Geometry check sheet. Reference: the model listing, model coordinates, mm. Face numbers are marked on the shaded views. A direction names the side the tool comes from. Coordinates: 2 decimals unless noted, no trailing zeros. Order: outer loops, then holes, each group sorted by start corner. A loop starts at its lowest first (then second) coordinate and runs counter-clockwise, first axis right, second up. Notation, with made-up numbers: (32.5, -18) - (63.5, -18) arc R8 cw to (63.5, -14) - close; hole circle Ø4 at (18.25, -2). An arc over 180 degrees is marked (long way). Use CSV: the item, a comma, the result in double quotes. Start each with the question number.
1) Sectioned sample at B-B, the plane y = 115. Record the cut outline in (x, z).
2) Depth check by flat-ended pin: P1, Ø8, axis at x = -19.5, y = 4, coming from the +Z side; P2, Ø3, axis at x = 4.5, y = 41.5, coming from the -Z side; P3, Ø9, axis at x = 35, z = -68.5, coming from the +Y side. Enter the tip coordinate at first touch or a pass-through.
3) Tool access check on the marked faces 1, 2 and 3. Record the directions out of +Z, -Z, +X, -X, +Y, -Y that give a thin tool (end or side, any length) a straight path to the whole face; none if there is none.
4) Sectioned sample at A-A, the plane x = 17.5. Record the cut outline in (y, z).
5) Thickness scan on probe 1 along Y at (x, z) = (5, -34.5); probe 2 along X at (y, z) = (208, -45.5); probe 3 along Z at (x, y) = (46, 44). Record the ranges inside material, lowest first. Write a range as [from, to].
6) Draft check along X on the marked faces 4, 5, 6 and 7. Enter one of: released by +X, released by -X, zero draft, split by the parting line, or undercut.
7) Sectioned sample at D-D, the plane x = 52.5. Record the cut outline in (y, z).
8) Sectioned sample at C-C, the plane x = 4.5. Record the cut outline in (y, z), and give its area (3 significant figures).
from build123d import *

# Parameters (mm, degrees)
ESQUISSE1_W             = 60
ESQUISSE1_H             = 60
BOSS_EXTRU_1_DEPTH      = 250
ESQUISSE2_W             = 40
ESQUISSE2_H             = 40
ENL_V_MAT_EXTRU_1_DEPTH = 250
ESQUISSE3_W             = 20
ESQUISSE3_H             = 41
ENL_V_MAT_EXTRU_7_DEPTH = 10
ESQUISSE4_W             = 60
ESQUISSE4_H             = 30
ESQUISSE4_W_2           = 30
ESQUISSE4_H_2           = 60
ESQUISSE4_H_3           = 30.275028017
BOSS_EXTRU_2_DEPTH      = 10
ESQUISSE6_R             = 2
ENL_V_MAT_EXTRU_8_DEPTH = 10


with BuildPart() as part:
    # Esquisse1 → Boss.-Extru.1 (new body)
    with BuildSketch(Plane(origin=(0, 0, 0), x_dir=(1, 0, 0), z_dir=(0, 1, 0))):
        with Locations((30, 30)):
            Rectangle(ESQUISSE1_W, ESQUISSE1_H)
    extrude(amount=BOSS_EXTRU_1_DEPTH)

    # Esquisse2 → Enlèv. mat.-Extru.1 (cut)
    with BuildSketch(Plane(origin=(0, 250, 0), x_dir=(1, 0, 0), z_dir=(0, 1, 0))):
        with Locations((30, 30)):
            Rectangle(ESQUISSE2_W, ESQUISSE2_H)
    extrude(amount=-ENL_V_MAT_EXTRU_1_DEPTH, mode=Mode.SUBTRACT)

    # Esquisse3 → Enlèv. mat.-Extru.7 (cut)
    with BuildSketch(Plane(origin=(0, 0, 0), x_dir=(0, 0, -1), z_dir=(1, 0, 0))):
        with Locations((30, 149.5)):
            Rectangle(ESQUISSE3_W, ESQUISSE3_H)
    extrude(amount=ENL_V_MAT_EXTRU_7_DEPTH, mode=Mode.SUBTRACT)

    # Esquisse4 → Boss.-Extru.2 (add)
    with BuildSketch(Plane(origin=(0, 0, 0), x_dir=(1, 0, 0), z_dir=(0, 1, 0))):
        with Locations((30, 75)):
            Rectangle(ESQUISSE4_W, ESQUISSE4_H)
        with Locations((-15, 30)):
            Rectangle(ESQUISSE4_W_2, ESQUISSE4_H_2)
        with Locations((75, 30)):
            Rectangle(ESQUISSE4_W_2, ESQUISSE4_H_2)
        with Locations((30, -15.137514009)):
            Rectangle(ESQUISSE4_W, ESQUISSE4_H_3)
    extrude(amount=BOSS_EXTRU_2_DEPTH)

    # Esquisse6 → Enlèv. mat.-Extru.8 (cut)
    with BuildSketch(Plane.ZY):
        with Locations((-34.5, 173.5)):
            Circle(ESQUISSE6_R)
        with Locations((-25.5, 173.5)):
            Circle(ESQUISSE6_R)
        with Locations((-34.5, 125.5)):
            Circle(ESQUISSE6_R)
        with Locations((-25.5, 125.5)):
            Circle(ESQUISSE6_R)
    extrude(amount=-ENL_V_MAT_EXTRU_8_DEPTH, mode=Mode.SUBTRACT)


solid = part.part
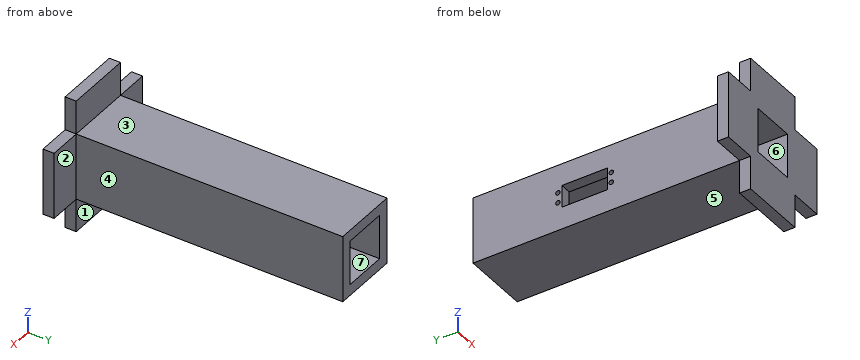
Evaluation:
1,outline,"(0, -60) - (60, -60) - (60, 0) - (0, 0) - close; hole (10, -50) - (50, -50) - (50, -10) - (10, -10) - close"
2,P1,"z = 0"
2,P2,"z = -60"
2,P3,"y = 10"
3,face 1,"-Z, +X, -X, +Y"
3,face 2,"+Z, -Z, +X, +Y"
3,face 3,"+Z, +X, -X, +Y"
4,outline,"(0, -90) - (10, -90) - (10, -60) - (250, -60) - (250, -50) - (0, -50) - close; (0, -10) - (250, -10) - (250, 0) - (10, 0) - (10, 30.28) - (0, 30.28) - close"
5,probe 1,"[0, 123.5], [127.5, 129], [170, 171.5], [175.5, 250]"
5,probe 2,"[0, 10], [50, 60]"
5,probe 3,"[-60, -50], [-10, 0]"
6,face 4,"released by +X"
6,face 5,"zero draft"
6,face 6,"undercut"
6,face 7,"undercut"
7,outline,"(0, -90) - (10, -90) - (10, -60) - (250, -60) - (250, 0) - (10, 0) - (10, 30.28) - (0, 30.28) - close"
8,outline,"(0, -90) - (10, -90) - (10, -60) - (250, -60) - (250, 0) - (10, 0) - (10, 30.28) - (0, 30.28) - close; hole circle Ø4 at (125.5, -34.5); hole circle Ø4 at (125.5, -25.5); hole (129, -40) - (170, -40) - (170, -20) - (129, -20) - close; hole circle Ø4 at (173.5, -34.5); hole circle Ø4 at (173.5, -25.5)"
8,area,"14,700 mm²"
